```python
from build123d import *

# Parameters (mm, degrees)
F0_W     = 101.6
F0_H     = 101.6
F1_DEPTH = 6.35
F2_W     = 76.2
F2_H     = 12.7
F3_DEPTH = 76.2
F5_D     = 6.35


with BuildPart() as f1:
    # F0 (on Top) → F1 (new body)
    with BuildSketch(Plane.XY):
        Rectangle(F0_W, F0_H)
    extrude(amount=F1_DEPTH)

    # F2 (on face) → F3 (join)
    with BuildSketch(Plane.XY.offset(6.35)):
        Rectangle(F2_W, F2_H)
    extrude(amount=F3_DEPTH)

    # F5 (through all)
    with Locations(Plane.XZ.offset(6.35)):
        with Locations((-12.7, 57.15), (12.7, 57.15)):
            Hole(F5_D / 2)


solid = f1.part
```
CAD build for the part. Positions are in the model's coordinates, mm. A direction names the side the tool comes from. Round coordinates to 2 decimals unless told otherwise and drop trailing zeros. Loops run counter-clockwise (first coordinate to the right, second up) from the corner with the lowest first, then second, coordinate; pieces in that order, holes last. Notation, with made-up numbers: M 7.25,26.25 L 33.25,26.25 A19 cw 33.25,38.25 Z; hole C 88.25,25.5 d2. An arc over 180 degrees is marked long. Use a Markdown table: item, result. Add a question column.
(1) Cut at A-A (z = 57.15). Give the cut face in (x, y) (3 decimals), and give its area (3 significant figures).
(2) Cut at B-B (x = 12.7). Give the cut face in (y, z) (3 decimals), and give its area (3 significant figures).
(3) Which spindle directions (+Z, -Z, +X, -X, +Y, -Y) get a long thin tool onto all of the face, cutting with end or side? Do faces 1 (the face through (38.1, 0, 44)), 2 (the face through (-1, 6.35, 44)), 3 (the face through (-1, -50.8, 3)), 4 (the face through (-38.1, 0, 44)), 5 (the face through (-50.8, -1, 3)). Say none if no direction does.
(4) Cut at C-C (y = 5). Give the cut face in (x, z) (3 decimals).
(5) Cut at D-D (x = -35). Give the cut face in (y, z).
(6) Flat gauge pins, fed straight in: pin 1 (10 mm diameter, centred on x = 12.7, z = 57.15, fed in from +Y); pin 2 (6 mm diameter, centred on x = -22.5, z = 43, fed in from -Y); pin 3 (14 mm diameter, centred on y = -2.5, z = 48.5, fed in from -X). Where does each tip first touch, or does it go through?
(7) Drill centre lines: line 1 (X direction, y = 1, z = 57); line 2 (Z direction, x = 12.7, y = 0.5) (3 decimals); line 3 (Y direction, x = -4, z = 67.5). Where is each one in solid material? Low to high.
(8) Pull direction Z, two halves, no side cores. Call faces 6 (the face through (13.39, 0.09, 54.05)), 7 (the face through (-12.01, 0.09, 54.05)), 8 (the face through (-1, 1, 0)), 9 (the face through (-1, -6.35, 44)): +Z half, -Z half, draft (parallel to the pull), parting line (faces both ways), or undercut.
Geometry says:
| question | item | result |
|---|---|---|
| 1 | outline | M -38.1,-6.35 L -15.875,-6.35 L -15.875,6.35 L -38.1,6.35 Z; M -9.525,-6.35 L 9.525,-6.35 L 9.525,6.35 L -9.525,6.35 Z; M 15.875,-6.35 L 38.1,-6.35 L 38.1,6.35 L 15.875,6.35 Z |
| 1 | area | 806 mm² |
| 2 | outline | M -50.8,0 L 50.8,0 L 50.8,6.35 L 6.35,6.35 L 6.35,53.975 L -6.35,53.975 L -6.35,6.35 L -50.8,6.35 Z; M -6.35,60.325 L 6.35,60.325 L 6.35,82.55 L -6.35,82.55 Z |
| 2 | area | 1,530 mm² |
| 3 | face 1 | +Z, +X, +Y, -Y |
| 3 | face 2 | +Z, +X, -X, +Y |
| 3 | face 3 | +Z, -Z, +X, -X, -Y |
| 3 | face 4 | +Z, -X, +Y, -Y |
| 3 | face 5 | +Z, -Z, -X, +Y, -Y |
| 4 | outline | M -50.8,0 L 50.8,0 L 50.8,6.35 L 38.1,6.35 L 38.1,82.55 L -38.1,82.55 L -38.1,6.35 L -50.8,6.35 Z; hole C -12.7,57.15 d6.35; hole C 12.7,57.15 d6.35 |
| 5 | outline | M -50.8,0 L 50.8,0 L 50.8,6.35 L 6.35,6.35 L 6.35,82.55 L -6.35,82.55 L -6.35,6.35 L -50.8,6.35 Z |
| 6 | pin 1 | stops at y = 6.35 |
| 6 | pin 2 | stops at y = -6.35 |
| 6 | pin 3 | stops at x = -38.1 |
| 7 | line 1 | x = -38.1 to -15.87, -9.53 to 9.53, 15.87 to 38.1 |
| 7 | line 2 | z = 0 to 53.975, 60.325 to 82.55 |
| 7 | line 3 | y = -6.35 to 6.35 |
| 8 | face 6 | undercut |
| 8 | face 7 | undercut |
| 8 | face 8 | -Z half |
| 8 | face 9 | draft |
